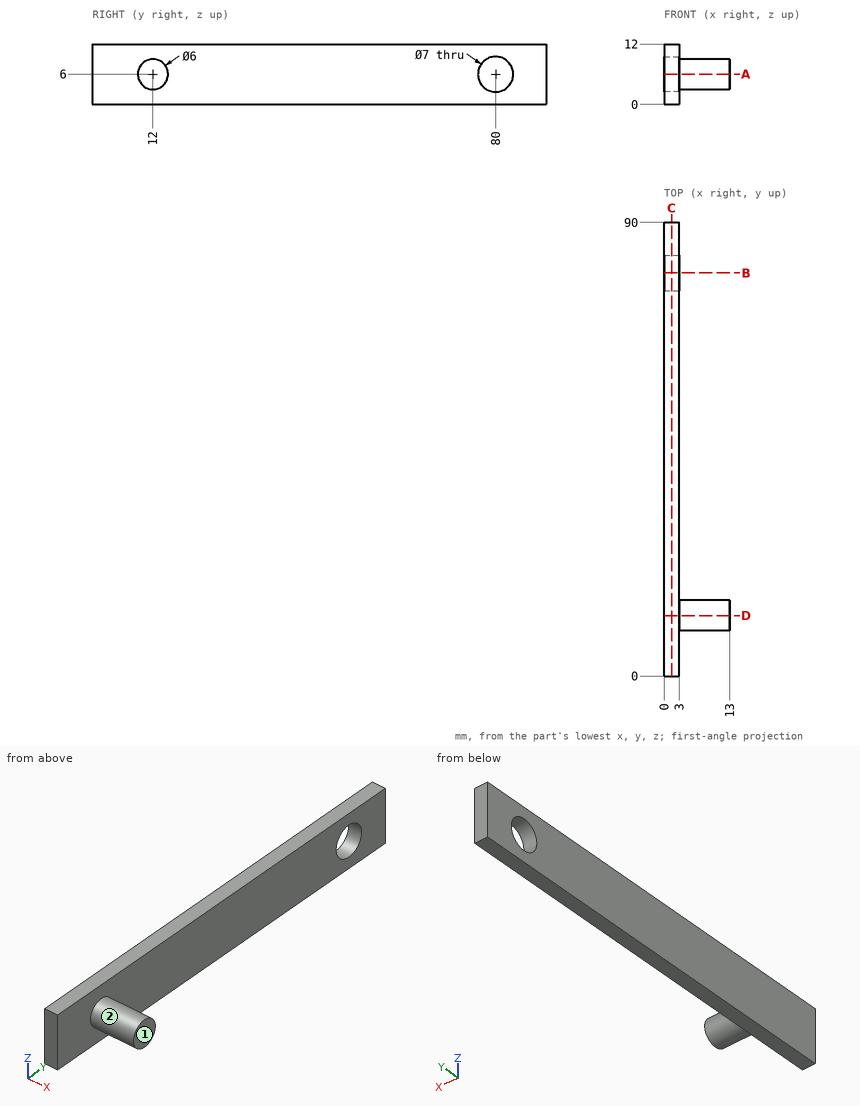
Design review of the part shown in the three views and the two pictorial views. Dimensions are in mm from the part's minimum x, y and z. A direction names the side the tool comes from. Round coordinates to 2 decimals unless told otherwise and drop trailing zeros. Loops run counter-clockwise (first coordinate to the right, second up) from the corner with the lowest first, then second, coordinate; pieces in that order, holes last. Notation, with made-up numbers: (85.25, -34) -> (135.25, -34) arc R33 ccw to (135.25, -4) -> close; hole circle Ø11 at (81.5, -31). An arc over 180 degrees is marked (long way). Return JSON: item names as keys, results as strings.
(1) Add section A-A on z = 6. Write out the cut boundary in (x, y).
Solved:
{"outline": "(0, 0) -> (3, 0) -> (3, 9) -> (13, 9) -> (13, 15) -> (3, 15) -> (3, 76.5) -> (0, 76.5) -> close; (0, 83.5) -> (3, 83.5) -> (3, 90) -> (0, 90) -> close"}
(2) Add section D-D on y = 12. Write out the cut boundary in (x, z).
Solved:
{"outline": "(0, 0) -> (3, 0) -> (3, 3) -> (13, 3) -> (13, 9) -> (3, 9) -> (3, 12) -> (0, 12) -> close"}
(3) For line 1 (Y direction, x = 0.95, z = 6); line 2 (X direction, y = 26.5, z = 6.5); line 3 (Y direction, x = 0.75, z = 4.5), list the stretches that pass through material, from the lowest coordinate up.
Solved:
{"line 1": "0 to 76.5, 83.5 to 90", "line 2": "0 to 3", "line 3": "0 to 76.84, 83.16 to 90"}
(4) For the marked faces 1 and 2, list the 3-axis set-ups (+Z, -Z, +X, -X, +Y, -Y) from which the entire face can be reached by the end or side of a thin tool; tool diameter is ignored.
Solved:
{"face 1": "+Z, -Z, +X, +Y, -Y", "face 2": "+X"}
(5) For pin 1 (5.5 mm diameter, centred on y = 80, z = 6, fed in from -X); pin 2 (5 mm diameter, centred on x = 4.5, z = 5, fed in from -Y); pin 3 (3 mm diameter, centred on x = 11, z = 9, fed in from -Y); pin 4 (3.5 mm diameter, centred on y = 53.5, z = 3, fed in from +X), all flat-tipped, find the tip position at first contact; note any pin that passes through.
Solved:
{"pin 1": "through", "pin 2": "y = 0", "pin 3": "y = 9.4", "pin 4": "x = 3"}
(6) Add section B-B on y = 80. Write out the cut boundary in (x, z).
Solved:
{"outline": "(0, 0) -> (3, 0) -> (3, 2.5) -> (0, 2.5) -> close; (0, 9.5) -> (3, 9.5) -> (3, 12) -> (0, 12) -> close"}
(7) Add section C-C on x = 1.5. Write out the cut boundary in (y, z).
Solved:
{"outline": "(0, 0) -> (90, 0) -> (90, 12) -> (0, 12) -> close; hole circle Ø7 at (80, 6)"}
